from build123d import *

# Parameters (mm, degrees)
SKETCH1_R           = 30
SKETCH1_R_2         = 3
SKETCH1_R_3         = 4.1
BOSS_EXTRUDE1_DEPTH = 5
FILLET1_R           = 0.5


with BuildPart() as part:
    # Sketch1 → Boss-Extrude1 (new body)
    with BuildSketch(Plane(origin=(0, 0, 0), x_dir=(0, 0, -1), z_dir=(1, 0, 0))):
        Circle(SKETCH1_R)
        with Locations((-25.5, 0)):
            Circle(SKETCH1_R_2, mode=Mode.SUBTRACT)
        Circle(SKETCH1_R_3, mode=Mode.SUBTRACT)
    extrude(amount=BOSS_EXTRUDE1_DEPTH)

    # Fillet1
    fillet1_edges = [part.edges().sort_by_distance(p)[0] for p in [
        (0, 0, 30),
        (5, 0, 30),
    ]]
    fillet(fillet1_edges, radius=FILLET1_R)


solid = part.part
Could you check a few things on this model? Use its own coordinates, in mm. Coordinates: 2 decimals unless noted, no trailing zeros. Order: outer loops, then holes, each group sorted by start corner. A loop starts at its lowest first (then second) coordinate and runs counter-clockwise, first axis right, second up. Notation, with made-up numbers: (71, -11) -> (112, -11) arc R22 cw to (112, 11) -> close; hole circle Ø10 at (82, 26.5). An arc over 180 degrees is marked (long way). One line per item, written item: value. Start each with the question number.
1) Imagine slicing it at B-B on z = 0. List the corners of the cut face in (x, y) for me.
2) If I drill on L1, parallel to Y at x = 3.2, z = 0; L2, parallel to Z at x = 3.4, y = 0.5; L3, parallel to Z at x = 1.5, y = -2, over which ranges is the centre line in solid material (lowest first)? Write a range as [from, to].
3) I'm going to push flat-ended pins straight in: pin 1 (1.5 mm diameter, centred on x = 2, y = 11, fed in from -Z); pin 2 (1 mm diameter, centred on x = 1, z = 11.5, fed in from +Y); pin 3 (2 mm diameter, centred on x = 3, z = -3, fed in from +Y); pin 4 (5 mm diameter, centred on y = 7, z = -2, fed in from -X). Where does each tip first touch, or does it pass through?
4) Imagine slicing it at C-C on x = 1.5. List the corners of the cut face in (y, z) for me, plus the area to 3 significant figures.
5) Imagine slicing it at A-A on y = 0. List the corners of the cut face in (x, z) for me.
6) We'd pull the mould along Y, two halves only. Please class faces 1 (the cylindrical face through (2.465, 4.065, 0.534)), 2 (the flat face through (5, 0, -6)), 3 (the cylindrical face through (2.47, 1.32, 29.97)): +Y half, -Y half, draft (parallel to the pull), parting line (faces both ways), or undercut.
Answer list:
1. outline: (0, -29.5) arc R0.5 ccw to (0.5, -30) -> (4.5, -30) arc R0.5 ccw to (5, -29.5) -> (5, -4.1) -> (0, -4.1) -> close; (0, 4.1) -> (5, 4.1) -> (5, 29.5) arc R0.5 ccw to (4.5, 30) -> (0.5, 30) arc R0.5 ccw to (0, 29.5) -> close
2. L1: y = [-30, -4.1], [4.1, 30]
2. L2: z = [-30, -4.07], [4.07, 22.54], [28.46, 30]
2. L3: z = [-29.93, -3.58], [3.58, 23.26], [27.74, 29.93]
3. pin 1: stops at z = -28.19
3. pin 2: stops at y = 27.91
3. pin 3: stops at y = 29.93
3. pin 4: stops at x = 0
4. outline: circle Ø60 at (0, 0); hole circle Ø8.2 at (0, 0); hole circle Ø6 at (0, 25.5)
4. area: 2,750 mm2
5. outline: (0, -29.5) arc R0.5 ccw to (0.5, -30) -> (4.5, -30) arc R0.5 ccw to (5, -29.5) -> (5, -4.1) -> (0, -4.1) -> close; (0, 4.1) -> (5, 4.1) -> (5, 22.5) -> (0, 22.5) -> close; (0, 28.5) -> (5, 28.5) -> (5, 29.5) arc R0.5 ccw to (4.5, 30) -> (0.5, 30) arc R0.5 ccw to (0, 29.5) -> close
6. face 1: undercut
6. face 2: draft
6. face 3: parting line
